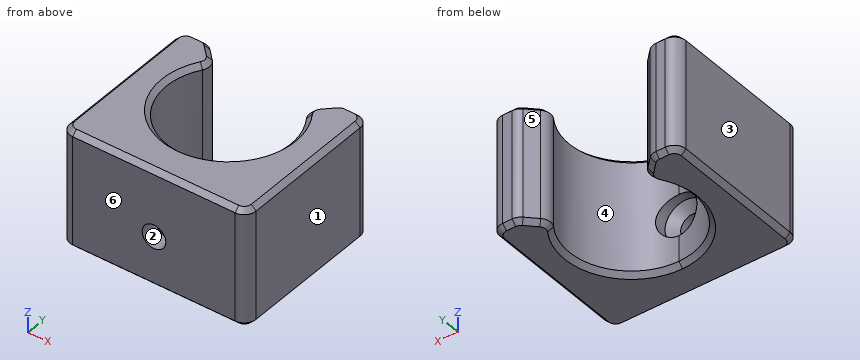
Autodesk Inventor part; units mm, degrees
ref_plane "YZ Plane" through (0, 0, 0) normal (1, 0, 0) x (0, 1, 0)
ref_plane "XZ Plane" through (0, 0, 0) normal (0, 1, 0) x (-1, 0, 0)
ref_plane "XY Plane" through (0, 0, 0) normal (0, 0, 1) x (1, 0, 0)
sketch "Sketch1" plane through (0, 0, 0) normal (0, 0, 1) x (1, 0, 0)
  arc A0 (0, 0) -> (7.8262, 17.5) centre (0, 10.5) ccw
  line L0 (0, 26.4) -> (0, -11.4)
  line L1 (-48.3956, 0) -> (48.6087, 0)
  line L2 (7.8262, 17.5) -> (11.3262, 21)
  line L3 (11.3262, 21) -> (15.75, 21)
  line L4 (15.75, 21) -> (15.75, -6)
  line L5 (15.75, -6) -> (0, -6)
  arc A1 (-7.8262, 17.5) -> (0, 0) centre (0, 10.5) ccw
  line L6 (48.3956, 0) -> (-48.6087, 0)
  line L7 (-7.8262, 17.5) -> (-11.3262, 21)
  line L8 (-11.3262, 21) -> (-15.75, 21)
  line L9 (-15.75, 21) -> (-15.75, -6)
  line L10 (-15.75, -6) -> (0, -6)
  dimension "d0" = 10.5
  dimension "d1" = 17.5
  dimension "d2" = 45
  dimension "d3" = 15.75
  dimension "d4" = 21
  dimension "d5" = 6
extrude "Extrusion1" add sketch "Sketch1" along normal blind 20
sketch "Sketch2" plane through (0, 0, 0) normal (0, 1, 0) x (-1, 0, 0)
  circle A0 centre (0, 8.6607) radius 2
  circle A1 centre (0, 8.6607) radius 3.5
  point P0 (0, 0)
  dimension "d8" = 7
  dimension "d9" = 4
extrude "Extrusion2" cut sketch "Sketch2" along normal through all both and the other way through all contours A0
extrude "Extrusion3" cut sketch "Sketch2" along normal blind 10 and the other way blind 3 contours A0 | A1
chamfer "Chamfer1" distance 1.5 angle 45 1 edges at (3.5, -3, 8.6607)
fillet "Fillet1" radius 2 8 edges at (-15.75, -6, 10) (15.75, -6, 10) (7.8262, 17.5, 10) (11.3262, 21, 10) (15.75, 21, 10) (-7.8262, 17.5, 10) (-11.3262, 21, 10) (-15.75, 21, 10)
chamfer "Chamfer2" distance 0.8 angle 45 32 edges at (-15.75, 7.5, 20) (-15.1642, -5.4142, 20) (0, -6, 20) (15.1642, -5.4142, 20) (15.75, 7.5, 20) (15.1642, 20.4142, 20) (12.9523, 21, 20) (11.3893, 20.8478, 20) (9.9007, 19.5745, 20) (8.486, 17.5284, 20) (0, 0, 20) (-8.486, 17.5284, 20) (-9.9007, 19.5745, 20) (-11.3893, 20.8478, 20) (-12.9523, 21, 20) (-15.1642, 20.4142, 20) (15.75, 7.5, 0) (15.1642, 20.4142, 0) (12.9523, 21, 0) (11.3893, 20.8478, 0) (9.9007, 19.5745, 0) (8.486, 17.5284, 0) (0, 0, 0) (-8.486, 17.5284, 0) (-9.9007, 19.5745, 0) (-11.3893, 20.8478, 0) (-12.9523, 21, 0) (-15.1642, 20.4142, 0) (-15.75, 7.5, 0) (-15.1642, -5.4142, 0) (0, -6, 0) (15.1642, -5.4142, 0)
equation "\"d1\" = 1.66667 * d0"
equation "\"d3\" = 1.5 * d0"
equation "\"d4\" = 2 * d0"
equation "\"D_Screw\" = 4"
equation "\"D_Screwhead\" = 6"
properties part number "_3DPrint"
Work out the finished part from the listing and answer in its coordinate system (mm). Face numbers are marked on the shaded views. A direction names the side the tool comes from. Give positions to 0.01 mm unless a question says otherwise; leave off trailing zeros. Write each loop counter-clockwise with the first axis right and the second up, starting at its lowest first coordinate (ties: lowest second). Pieces come first, ordered by that corner, then holes.
(1) The part is cut by section A-A on z = 17. Write down the section's boundary in (x, y), plus the area to 3 significant figures.
Final values:
outline: (-15.75, -4) arc R2 ccw to (-13.75, -6) - (13.75, -6) arc R2 ccw to (15.75, -4) - (15.75, 19) arc R2 ccw to (13.75, 21) - (12.15, 21) arc R2 ccw to (10.74, 20.41) - (9.06, 18.73) arc R2 ccw to (8.8, 16.23) arc R10.5 cw to (0, 0) arc R10.5 cw to (-8.8, 16.23) arc R2 ccw to (-9.06, 18.73) - (-10.74, 20.41) arc R2 ccw to (-12.15, 21) - (-13.75, 21) arc R2 ccw to (-15.75, 19) - close
area: 470 mm2
(2) Straight lines are drawn through the part: line 1 (Z direction, x = 0, y = -5.15); line 2 (Y direction, x = 3.5, z = 1); line 3 (X direction, y = 18, z = 13). For each, find the intervals that lie inside material, in ascending order.
Final values:
line 1: z = 0 to 6.66, 10.66 to 20
line 2: y = -6 to 0.6
line 3: x = -15.75 to -8.59, 8.59 to 15.75
(3) The mould has two halves that part along X. Classify the marked faces 1, 2 and 3: pulls with the +X half, pulls with the -X half, needs draft (parallel to the pull), parting line crosses it, or undercut.
Final values:
face 1: pulls with the +X half
face 2: undercut
face 3: pulls with the -X half
(4) Flat-ended cylindrical pins translate along their axes: pin 1 Ø3 at (x, z) = (-9.5, 13) entering from +Y; pin 2 Ø9 at (x, z) = (0, 8.66) entering from +Y. Find the tip coordinate at first contact, or state that the pin passes through.
Final values:
pin 1: stops at y = 20.63
pin 2: stops at y = 1.01
(5) Which of the six approach directions +Z, -Z, +X, -X, +Y, -Y give full straight-line access (tool end or side, diameter ignored) to the marked faces 4, 5 and 6?
Final values:
face 4: +Z, -Z
face 5: +Z, -Z, +Y
face 6: +Z, -Z, +X, -X, -Y
